Could you check a few things on this model? Use its own coordinates, in mm. Face numbers are marked on the shaded views. A direction names the side the tool comes from. Coordinates: 2 decimals unless noted, no trailing zeros. Order: outer loops, then holes, each group sorted by start corner. A loop starts at its lowest first (then second) coordinate and runs counter-clockwise, first axis right, second up. Notation, with made-up numbers: (-5.75, 67) -> (10.25, 67) arc R21 ccw to (10.25, 96) -> close; hole circle Ø9 at (-8, 40). An arc over 180 degrees is marked (long way). Return JSON: item names as keys, results as strings. Group by question number.
Autodesk Inventor part; units mm, degrees
ref_plane "YZ Plane" through (0, 0, 0) normal (1, 0, 0) x (0, 1, 0)
ref_plane "XZ Plane" through (0, 0, 0) normal (0, 1, 0) x (-1, 0, 0)
ref_plane "XY Plane" through (0, 0, 0) normal (0, 0, 1) x (1, 0, 0)
sketch "スケッチ1" plane through (0, 0, 0) normal (0, 1, 0) x (-1, 0, 0)
  line L0 (30, 4) -> (30, -26)
  line L1 (30, -26) -> (-30, -26)
  line L2 (-30, -26) -> (-30, 4)
  line L3 (28, 4) -> (28, -24)
  line L4 (28, -24) -> (-28, -24)
  line L5 (-28, -24) -> (-28, 4)
  line L6 (-30, 4) -> (-28, 4)
  line L7 (28, 4) -> (30, 4)
  point P0 (0, 0)
  dimension "d0" = 60
  dimension "d2" = 30
  dimension "d3" = 28
  dimension "d4" = 56
  dimension "d5" = 28
  dimension "d6" = 24
  dimension "d7" = 30
  dimension "d8" = 26
  dimension "d9" = 28
  dimension "d11" = 28
extrude "押し出し1" add sketch "スケッチ1" along normal blind 30
sketch "スケッチ2" plane through (30, 0, 4) normal (1, 0, 0) x (0, 0, -1)
  line L0 (30, 0) -> (30, 30)
  line L1 (0, 0) -> (0, 30)
  line L2 (30, 30) -> (0, 25)
  line L3 (30, 0) -> (0, 5)
  point P0 (4, 0)
  dimension "d75" = 20
extrude "押し出し2" cut sketch "スケッチ2" against normal blind 60 keep common part
sketch "スケッチ3" plane through (30, 0, -26) normal (1, 0, 0) x (0, 0, -1)
  line L0 (-30, 5) -> (-30, 25)
  line L1 (0, 0) -> (0, 30)
  arc A0 (-27, 11) -> (-27, 19) centre (-27, 15) ccw
  line L2 (-27, 19) -> (-30, 19)
  line L3 (-27, 11) -> (-30, 11)
  point P0 (-26, 0)
  dimension "d20" = 8
  dimension "d79" = 3
  dimension "d82" = 15
extrude "押し出し3" cut sketch "スケッチ3" against normal blind 2
sketch "スケッチ4" plane through (-30, 0, -26) normal (-1, 0, 0) x (0, 0, 1)
  line L0 (30, 5) -> (30, 25)
  arc A0 (27, 20) -> (27, 10) centre (27, 15) ccw
  line L1 (27, 20) -> (30, 20)
  line L2 (27, 10) -> (30, 10)
  point P0 (26, 0)
  point P1 (0, 30)
  dimension "d25" = 10
  dimension "d80" = 3
  dimension "d81" = 15
extrude "押し出し4" cut sketch "スケッチ4" against normal blind 2
sketch "スケッチ7" plane through (30, 0, -26) normal (0, 0, -1) x (-1, 0, 0)
  line L0 (0, 0) -> (60, 0)
  line L1 (0, 0) -> (0, 30)
  circle A0 centre (30, 15) radius 5
  point P0 (30, 0)
  dimension "d45" = 10
  dimension "d47" = 15
  dimension "d48" = 30
hole "穴2" at (0, 15, -26) direction (0, 0, 1) diameter 10 end through all
sketch "スケッチ8" plane through (30, 0, -26) normal (0, 0, -1) x (-1, 0, 0)
  circle A0 centre (30, 15) radius 5
  line L0 (0, 0) -> (0, 30)
  circle A1 centre (30, 22) radius 1
  line L1 (30, 15) -> (30, 22)
  point P0 (30, 0)
  dimension "d56" = 2
  dimension "d58" = 0
  dimension "d62" = 7
hole "穴3" at (0, 22, -26) direction (0, 0, 1) diameter 2 end through all
pattern_circular "円形状パターン2" count 8 over 360 about axis through (0, 15, 47.4847) along (0, 0, -1) of "穴2", "穴3"
sketch "スケッチ9" plane through (30, 0, -26) normal (1, 0, 0) x (0, 0, -1)
  arc A0 (-27, 11) -> (-27, 19) centre (-27, 15) ccw
  line L0 (-30, 19) -> (-30, 25)
  circle A1 centre (-27, 22) radius 1
  line L1 (-27, 15) -> (-27, 22)
  point P0 (-26, 0)
  dimension "d83" = 2
  dimension "d85" = 7
hole "穴4" at (30, 22, 1) direction (-1, 0, 0) diameter 2 end through all
pattern_circular "円形状パターン3" count 5 over 180 about axis through (30, 15, 1) along (-1, 0, 0) of "穴4"
sketch "スケッチ10" plane through (30, 0, -26) normal (0, 0, -1) x (-1, 0, 0)
  circle A0 centre (30, 15) radius 5
  line L0 (0, 30) -> (60, 30)
  circle A1 centre (15, 26) radius 1.65
  circle A2 centre (15, 4) radius 1.65
  circle A3 centre (45, 4) radius 1.65
  circle A4 centre (45, 26) radius 1.65
  point P0 (30, 0)
  dimension "d96" = 30
  dimension "d98" = 22
  dimension "d99" = 4
  dimension "d100" = 22
  dimension "d101" = 4
  dimension "d102" = 30
  dimension "d103" = 15
  dimension "d104" = 15
  dimension "d105" = 3.3
hole "穴5" at (15, 4, -26) at (-15, 4, -26) at (-15, 26, -26) at (15, 26, -26) direction (0, 0, 1) diameter 3.3 end through all
properties part number "12" material "アルミニウム 6061"
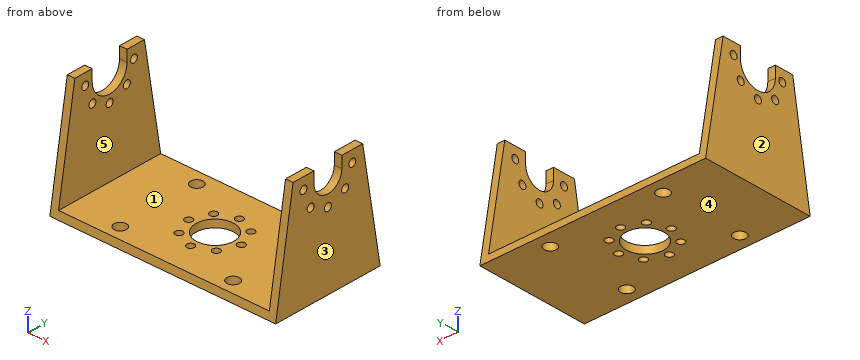
Q1. We'd pull the mould along X, two halves only. Please class the marked faces 3, 4 and 5: pulls with the +X half, pulls with the -X half, needs draft (parallel to the pull), parting line crosses it, or undercut.
Q2. I need wall thicknesses on line 1 along X through (y, z) = (4, -25.5); line 2 along X through (y, z) = (11.25, -19.5); line 3 along Y through (x, z) = (29, 1). Which ranges of each line are inside material? Lowest first, please. Write a range as from..to.
Q3. On a 3-axis mill with a long thin cutter (end or side, diameter ignored), from which of +Z, -Z, +X, -X, +Y, -Y can I reach the whole of each face in a straight line? I mean the marked faces 1 and 2. Say none if no direction works.
Q4. I want a section at B-B on x = 0. Please give me the cut outline in (y, z).
Q5. I want a section at A-A on z = -20. Please give me the cut outline in (x, y).
Q6. I want a section at D-D on x = -7. Please give me the cut outline in (y, z).
Q7. I'm going to push flat-ended pins straight in: pin 1 Ø10 at (x, y) = (-22, 3.5) entering from +Z; pin 2 Ø1.6 at (x, z) = (29.5, 2) entering from +Y; pin 3 Ø12 at (x, z) = (22.5, -5.5) entering from -Y. Where does each tip first touch, or does it pass through?
Q8. I want a section at C-C on y = 8. Please give me the cut outline in (x, z), and give its area (3 significant figures).
Response values:
{
 "1": {"face 3": "pulls with the +X half", "face 4": "needs draft", "face 5": "undercut"},
 "2": {"line 1": "x = -30..-16.65, -13.35..13.35, 16.65..30", "line 2": "x = -30..-28, 28..30", "line 3": "y = 4.5..7, 9..11, 19..21, 23..25.5"},
 "3": {"face 1": "+Z, +Y, -Y", "face 2": "+Z, -Z, -X, +Y, -Y"},
 "4": {"outline": "(0, -26) -> (7, -26) -> (7, -24) -> (0.33, -24) -> close; (9, -26) -> (10, -26) -> (10, -24) -> (9, -24) -> close; (20, -26) -> (21, -26) -> (21, -24) -> (20, -24) -> close; (23, -26) -> (30, -26) -> (29.67, -24) -> (23, -24) -> close"},
 "5": {"outline": "(-30, 1) -> (-28, 1) -> (-28, 29) -> (-30, 29) -> close; (28, 1) -> (30, 1) -> (30, 29) -> (28, 29) -> close"},
 "6": {"outline": "(0, -26) -> (14, -26) -> (14, -24) -> (0.33, -24) -> close; (16, -26) -> (30, -26) -> (29.67, -24) -> (16, -24) -> close"},
 "7": {"pin 1": "stops at z = -24", "pin 2": "stops at y = 25.47", "pin 3": "stops at y = 3.02"},
 "8": {"outline": "(-30, -26) -> (-1, -26) -> (-1, -24) -> (-28, -24) -> (-28, 0) -> (-30, 0) -> close; (-30, 2) -> (-28, 2) -> (-28, 4) -> (-30, 4) -> close; (1, -26) -> (30, -26) -> (30, 0) -> (28, 0) -> (28, -24) -> (1, -24) -> close; (28, 2) -> (30, 2) -> (30, 4) -> (28, 4) -> close", "area": "220 mm²"}
}
